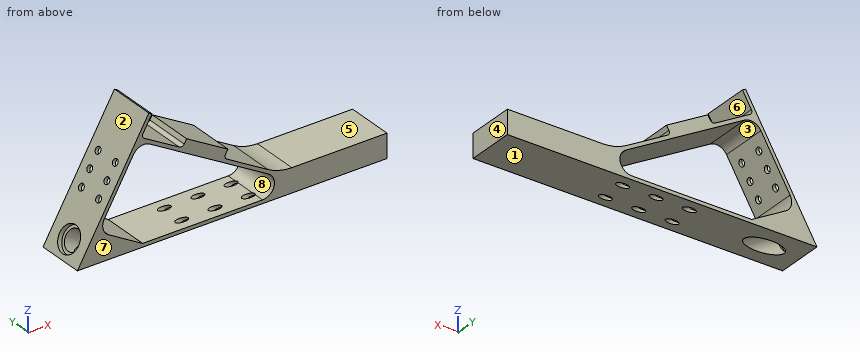
```python
from build123d import *

# Parameters (mm, degrees)
F1_DEPTH = 10
F3_DEPTH = 20
F4_R     = 4.25
F5_DEPTH = 112.584302492
F4_R_2   = 5.5
F6_DEPTH = 2
F4_R_3   = 1.395
F7_DEPTH = 112.584302492


with BuildPart() as f1:
    # F0 (on Front) → F1 (new body, symmetric)
    with BuildSketch(Plane.XZ):
        with BuildLine():
            Line((30, 51.9615242271), (0, 0))
            Line((0, 0), (130, 0))
            Line((130, 0), (130, 10))
            Line((130, 10), (90.0384757729, 10))
            ThreePointArc((90.0384757729, 10), (84.8620948709, 10.6814834742), (80.0384757729, 12.6794919243))
            Line((80.0384757729, 12.6794919243), (62.7390923627, 22.667295593))
            ThreePointArc((62.7390923627, 22.667295593), (62.0402036233, 23.578105131), (62.1900542571, 24.7163336987))
            Line((62.1900542571, 24.7163336987), (63.1900542571, 26.4483845063))
            Line((63.1900542571, 26.4483845063), (45.8695461814, 36.4483845063))
            Line((45.8695461814, 36.4483845063), (44.8695461814, 34.7163336987))
            ThreePointArc((44.8695461814, 34.7163336987), (43.9587366433, 34.0174449592), (42.8205080757, 34.167295593))
            Line((42.8205080757, 34.167295593), (28.0980762114, 42.667295593))
            ThreePointArc((28.0980762114, 42.667295593), (27.3991874719, 43.578105131), (27.5490381057, 44.7163336987))
            Line((27.5490381057, 44.7163336987), (31.2990381057, 51.2115242271))
            Line((31.2990381057, 51.2115242271), (30, 51.9615242271))
        make_face()
    extrude(amount=F1_DEPTH, both=True)

    # F2 (on face) → F3 (cut)
    with BuildSketch(Plane.XZ.offset(10)):
        with BuildLine():
            ThreePointArc((30.3791651246, 39.6182574873), (26.5850698991, 40.1177595999), (23.5490381057, 37.7881304684))
            Line((23.5490381057, 37.7881304684), (11.2990381057, 16.5705080757))
            ThreePointArc((11.2990381057, 16.5705080757), (10.7995359932, 12.7764128502), (13.1291651246, 9.7403810568))
            Line((13.1291651246, 9.7403810568), (27.4019237886, 1.5))
            Line((27.4019237886, 1.5), (77.7416697508, 1.5))
            ThreePointArc((77.7416697508, 1.5), (82.5712988822, 5.2059047745), (80.2416697508, 10.8301270189))
            Line((80.2416697508, 10.8301270189), (30.3791651246, 39.6182574873))
        make_face()
    extrude(amount=-F3_DEPTH, mode=Mode.SUBTRACT)

    # F4 (on face) → F5 (cut, through all)
    with BuildSketch(Plane(origin=(0, 0, 0), x_dir=(0, -1, 0), z_dir=(-0.8660254038, 0, 0.5))):
        with Locations((0, 7.5)):
            Circle(F4_R)
    extrude(amount=-F5_DEPTH, mode=Mode.SUBTRACT)

    # F4 (on face) → F6 (cut)
    with BuildSketch(Plane(origin=(0, 0, 0), x_dir=(0, -1, 0), z_dir=(-0.8660254038, 0, 0.5))):
        with Locations((0, 7.5)):
            Circle(F4_R_2)
        with Locations((0, 7.5)):
            Circle(F4_R, mode=Mode.SUBTRACT)
    extrude(amount=-F6_DEPTH, mode=Mode.SUBTRACT)

    # F4 (on face) → F7 (cut, through all)
    with BuildSketch(Plane(origin=(0, 0, 0), x_dir=(0, -1, 0), z_dir=(-0.8660254038, 0, 0.5))):
        with Locations((-5, 25)):
            Circle(F4_R_3)
        with Locations((5, 32)):
            Circle(F4_R_3)
        with Locations((-5, 32)):
            Circle(F4_R_3)
        with Locations((5, 39)):
            Circle(F4_R_3)
        with Locations((-5, 39)):
            Circle(F4_R_3)
        with Locations((5, 25)):
            Circle(F4_R_3)
    extrude(amount=-F7_DEPTH, mode=Mode.SUBTRACT)


solid = f1.part
```
Can you work these out from the model? Positions are in its coordinate system, mm. Face numbers are marked on the shaded views. A direction names the side the tool comes from. Round coordinates to 2 decimals unless told otherwise and drop trailing zeros. Loops run counter-clockwise (first coordinate to the right, second up) from the corner with the lowest first, then second, coordinate; pieces in that order, holes last. Notation, with made-up numbers: M 5.5,39.25 L 55.5,39.25 A10 cw 55.5,47.25 Z; hole C 2,-35 d3. An arc over 180 degrees is marked long. Answer as a JSON object with one key per item and string values. Group by question number.
Q1. Will these pins go through, and if not, where does the flat tip stop? pin 1 (1.5 mm diameter, centred on x = 106, y = -7.5, fed in from +Z); pin 2 (10 mm diameter, centred on x = 40, y = -1.5, fed in from +Z).
Q2. Imagine slicing it at C-C, the plane y = 2. Count the separate pieces of the cut face and the enclosed holes in it, then the cut area to 3 significant figures.
Q3. Imagine slicing it at D-D, the plane x = 119. Please give me the cut outline in (y, z).
Q4. On a 3-axis mill with a long thin cutter (end or side, diameter ignored), from which of +Z, -Z, +X, -X, +Y, -Y can I reach the whole of each face in a straight line? I mean the marked faces 5, 6, 7 and 8. Say none if no direction works.
Q5. We'd pull the mould along X, two halves only. Please class the marked faces 1, 2, 3 and 4: +X half, -X half, draft (parallel to the pull), parting line (faces both ways), or undercut.
Q6. Imagine slicing it at B-B, the plane x = 55.5. Please give me the cut outline in (y, z).
Q7. Imagine slicing it at A-A, the plane y = 8.25. Please give me the cut outline in (x, z).
Q8. Please list where these lines run through material, in increasing order: L1, parallel to X at y = 8.75, z = 35; L2, parallel to Z at x = 57, y = 0.25; L3, parallel to Z at x = 95.5, y = 2.5.
Findings:
{
 "1": {"pin 1": "stops at z = 10", "pin 2": "stops at z = 38.68"},
 "2": {"separate pieces": "2", "enclosed holes": "1", "area": "903 mm2"},
 "3": {"outline": "M -10,0 L 10,0 L 10,10 L -10,10 Z"},
 "4": {"face 5": "+Z, +X, +Y, -Y", "face 6": "+X, +Y, -Y", "face 7": "+Z, -Z, +X, -X, -Y", "face 8": "+Y, -Y"},
 "5": {"face 1": "draft", "face 2": "-X half", "face 3": "undercut", "face 4": "+X half"},
 "6": {"outline": "M -10,0 L 10,0 L 10,1.5 L -10,1.5 Z; M -10,25.11 L 10,25.11 L 10,30.89 L -10,30.89 Z"},
 "7": {"outline": "M 0,0 L 130,0 L 130,10 L 90.04,10 A20 cw 80.04,12.68 L 62.74,22.67 A1.5 cw 62.19,24.72 L 63.19,26.45 L 45.87,36.45 L 44.87,34.72 A1.5 cw 42.82,34.17 L 28.1,42.67 A1.5 cw 27.55,44.72 L 31.3,51.21 L 30,51.96 Z; hole M 11.3,16.57 A5 ccw 13.13,9.74 L 27.4,1.5 L 77.74,1.5 A5 ccw 80.24,10.83 L 30.38,39.62 A5 ccw 23.55,37.79 Z"},
 "8": {"L1": "x = 20.21 to 21.94, 38.38 to 41.38, 45.03 to 48.38", "L2": "z = 0 to 1.5, 24.25 to 30.02", "L3": "z = 0 to 10"}
}
